The listing builds one solid part. Answer for the finished solid, in the listing's coordinates (mm). Round coordinates to 2 decimals unless told otherwise and drop trailing zeros. Loops run counter-clockwise (first coordinate to the right, second up) from the corner with the lowest first, then second, coordinate; pieces in that order, holes last. Notation, with made-up numbers: M 60,-25.5 L 107,-25.5 A19 cw 107,-2.5 Z; hole C 86.5,-9.5 d2. An arc over 180 degrees is marked long. Answer as a JSON object with one key per item and string values.
```python
from build123d import *

# Parameters (mm, degrees)
SKETCH1_R           = 2.1
BOSS_EXTRUDE1_DEPTH = 16


with BuildPart() as part:
    # Sketch1 → Boss-Extrude1 (new body)
    with BuildSketch(Plane.XY):
        with BuildLine():
            Line((-4, 0), (-4, 30.2))
            ThreePointArc((-4, 30.2), (-2.141570433, 33.578413249), (1.706838041, 33.817554962))
            ThreePointArc((1.706838041, 33.817554962), (12.05, 31.5), (22.393161959, 33.817554962))
            ThreePointArc((22.393161959, 33.817554962), (26.241570433, 33.578413249), (28.1, 30.2))
            Line((28.1, 30.2), (28.1, 0))
            ThreePointArc((28.1, 0), (26.241570433, -3.378413249), (22.393161959, -3.617554962))
            ThreePointArc((22.393161959, -3.617554962), (12.05, -1.3), (1.706838041, -3.617554962))
            ThreePointArc((1.706838041, -3.617554962), (-2.141570433, -3.378413249), (-4, 0))
        make_face()
        Circle(SKETCH1_R, mode=Mode.SUBTRACT)
        with Locations((0, 30.2)):
            Circle(SKETCH1_R, mode=Mode.SUBTRACT)
        with Locations((24.1, 30.2)):
            Circle(SKETCH1_R, mode=Mode.SUBTRACT)
        with Locations((24.1, 0)):
            Circle(SKETCH1_R, mode=Mode.SUBTRACT)
    extrude(amount=BOSS_EXTRUDE1_DEPTH)


solid = part.part
```
Item 1: The part is cut by section C-C (x = 13.5). Give the vertices of the cut face in (y, z), then the cut area to 3 significant figures.
Values follow:
{"outline": "M -1.34,0 L 31.54,0 L 31.54,16 L -1.34,16 Z", "area": "526 mm^2"}
Item 2: Determine the mould class of faces 1 (the face through (26.289, -3.348, 7.888)), 2 (the face through (-4, 15, 8)), 3 (the face through (12, 15, 16)) for opening direction X: released by +X, released by -X, zero draft, split by the parting line, or undercut.
Values follow:
{"face 1": "undercut", "face 2": "released by -X", "face 3": "zero draft"}
Item 3: Straight lines are drawn through the part: line 1 (Y direction, x = 24.1, z = 12.75); line 2 (Y direction, x = 23.5, z = 14); line 3 (X direction, y = 28.5, z = 9). For each, find the intervals that lie inside material, in ascending order.
Values follow:
{"line 1": "-4 to -2.1, 2.1 to 28.1, 32.3 to 34.2", "line 2": "-3.95 to -2.01, 2.01 to 28.19, 32.21 to 34.15", "line 3": "-4 to -1.23, 1.23 to 22.87, 25.33 to 28.1"}
Item 4: The part is cut by section B-B (x = 24.1). Give the vertices of the cut face in (y, z), then the cut area to 3 significant figures.
Values follow:
{"outline": "M -4,0 L -2.1,0 L -2.1,16 L -4,16 Z; M 2.1,0 L 28.1,0 L 28.1,16 L 2.1,16 Z; M 32.3,0 L 34.2,0 L 34.2,16 L 32.3,16 Z", "area": "477 mm^2"}
Item 5: Flat-ended cylindrical pins translate along their axes: P1, Ø2, axis at x = 18, y = 30.5, coming from the -Z side; P2, Ø8, axis at x = 6.5, z = 6, coming from the -Y side; P3, Ø5, axis at x = 6, z = 6, coming from the -Y side. Find the tip coordinate at first contact, or state that the pin passes through.
Values follow:
{"P1": "z = 0", "P2": "y = -3.26", "P3": "y = -2.86"}
Item 6: The part is cut by section A-A (z = 7.25). Give the vertices of the cut face in (x, y).
Values follow:
{"outline": "M -4,0 A4 ccw 1.71,-3.62 A24.24 cw 22.39,-3.62 A4 ccw 28.1,0 L 28.1,30.2 A4 ccw 22.39,33.82 A24.24 cw 1.71,33.82 A4 ccw -4,30.2 Z; hole C 0,0 d4.2; hole C 0,30.2 d4.2; hole C 24.1,0 d4.2; hole C 24.1,30.2 d4.2"}
